```python
from build123d import *

# Parameters (mm, degrees)
SKETCH1_W            = 28
SKETCH1_H            = 45
BOSS_EXTRUDE1_DEPTH  = 7
SKETCH7_W            = 4
SKETCH7_H            = 7
BOSS_EXTRUDE2_DEPTH  = 6
SKETCH6_W            = 4
SKETCH6_H            = 7
BOSS_EXTRUDE3_DEPTH  = 6
SKETCH10_R           = 1
CUT_EXTRUDE1_DEPTH   = 6
SKETCH11_W           = 24
SKETCH11_H           = 5
CUT_EXTRUDE2_DEPTH   = 43
SKETCH16_W           = 36
SKETCH16_H           = 2
BOSS_EXTRUDE7_DEPTH  = 2
SKETCH17_W           = 36
SKETCH17_H           = 2
BOSS_EXTRUDE8_DEPTH  = 2
SKETCH30_W           = 40
SKETCH30_H           = 12
BOSS_EXTRUDE13_DEPTH = 11
SKETCH31_W           = 24
SKETCH31_H           = 10
CUT_EXTRUDE11_DEPTH  = 10
SKETCH32_W           = 24
SKETCH32_H           = 5
CUT_EXTRUDE12_DEPTH  = 1
SKETCH33_R           = 1
CUT_EXTRUDE13_DEPTH  = 11
SKETCH34_R           = 1
CUT_EXTRUDE14_DEPTH  = 11


with BuildPart() as part:
    # Sketch1 → Boss-Extrude1 (new body)
    with BuildSketch(Plane(origin=(0, 0, 0), x_dir=(1, 0, 0), z_dir=(0, 1, 0))):
        with Locations((14, 22.5)):
            Rectangle(SKETCH1_W, SKETCH1_H)
    extrude(amount=BOSS_EXTRUDE1_DEPTH)

    # Sketch7 → Boss-Extrude2 (add)
    with BuildSketch(Plane(origin=(28, 0, 0), x_dir=(0, 0, -1), z_dir=(1, 0, 0))):
        with Locations((43, 3.5)):
            Rectangle(SKETCH7_W, SKETCH7_H)
    extrude(amount=BOSS_EXTRUDE2_DEPTH)

    # Sketch6 → Boss-Extrude3 (add)
    with BuildSketch(Plane.ZY):
        with Locations((-43, 3.5)):
            Rectangle(SKETCH6_W, SKETCH6_H)
    extrude(amount=BOSS_EXTRUDE3_DEPTH)

    # Sketch10 → Cut-Extrude1 (cut)
    with BuildSketch(Plane.XY.offset(-41)):
        with Locations((-4, 2)):
            Circle(SKETCH10_R)
        with Locations((32, 2)):
            Circle(SKETCH10_R)
    extrude(amount=-CUT_EXTRUDE1_DEPTH, mode=Mode.SUBTRACT)

    # Sketch11 → Cut-Extrude2 (cut)
    with BuildSketch(Plane(origin=(0, 0, -45), x_dir=(-1, 0, 0), z_dir=(0, 0, -1))):
        with Locations((-14, 3.5)):
            Rectangle(SKETCH11_W, SKETCH11_H)
    extrude(amount=-CUT_EXTRUDE2_DEPTH, mode=Mode.SUBTRACT)

    # Sketch16 → Boss-Extrude7 (add)
    with BuildSketch(Plane.ZY):
        with Locations((-23, 4)):
            Rectangle(SKETCH16_W, SKETCH16_H)
    extrude(amount=BOSS_EXTRUDE7_DEPTH)

    # Sketch17 → Boss-Extrude8 (add)
    with BuildSketch(Plane(origin=(28, 0, 0), x_dir=(0, 0, -1), z_dir=(1, 0, 0))):
        with Locations((23, 4)):
            Rectangle(SKETCH17_W, SKETCH17_H)
    extrude(amount=BOSS_EXTRUDE8_DEPTH)

    # Sketch30 → Boss-Extrude13 (add)
    with BuildSketch(Plane(origin=(0, 0, -45), x_dir=(-1, 0, 0), z_dir=(0, 0, -1))):
        with Locations((-14, 3.5)):
            Rectangle(SKETCH30_W, SKETCH30_H)
    extrude(amount=BOSS_EXTRUDE13_DEPTH)

    # Sketch31 → Cut-Extrude11 (cut)
    with BuildSketch(Plane(origin=(0, 0, -56), x_dir=(-1, 0, 0), z_dir=(0, 0, -1))):
        with Locations((-14, 3.5)):
            Rectangle(SKETCH31_W, SKETCH31_H)
    extrude(amount=-CUT_EXTRUDE11_DEPTH, mode=Mode.SUBTRACT)

    # Sketch32 → Cut-Extrude12 (cut)
    with BuildSketch(Plane(origin=(0, 0, -46), x_dir=(-1, 0, 0), z_dir=(0, 0, -1))):
        with Locations((-14, 3.5)):
            Rectangle(SKETCH32_W, SKETCH32_H)
    extrude(amount=-CUT_EXTRUDE12_DEPTH, mode=Mode.SUBTRACT)

    # Sketch33 → Cut-Extrude13 (cut)
    with BuildSketch(Plane.XY.offset(-45)):
        with Locations((32, 2)):
            Circle(SKETCH33_R)
    extrude(amount=-CUT_EXTRUDE13_DEPTH, mode=Mode.SUBTRACT)

    # Sketch34 → Cut-Extrude14 (cut)
    with BuildSketch(Plane.XY.offset(-45)):
        with Locations((-4, 2)):
            Circle(SKETCH34_R)
    extrude(amount=-CUT_EXTRUDE14_DEPTH, mode=Mode.SUBTRACT)


solid = part.part
```
Design review of the part built by this model. Coordinates are the model's own, in mm. A direction names the side the tool comes from. Coordinates: 2 decimals unless noted, no trailing zeros. Write each loop counter-clockwise with the first axis right and the second up, starting at its lowest first coordinate (ties: lowest second). Pieces come first, ordered by that corner, then holes. Notation, with made-up numbers: M 38,19.5 L 47,19.5 A23 ccw 47,56.5 Z; hole C 79,-22.75 d3. An arc over 180 degrees is marked long. Answer as a JSON object with one key per item and string values.
Item 1: Machinability: for faces 1 (the flat face through (-1, 3, -23)), 2 (the flat face through (26, 3, -35)), 3 (the flat face through (14, -1, -45)), 4 (the flat face through (30, 4, -23)), 5 (the flat face through (-1, 4, -5)), which of the approach directions +Z, -Z, +X, -X, +Y, -Y give a long, thin tool a straight path to every point of the face, cutting with its end or side? Answer none if there is none.
Outcome:
{"face 1": "+Z, -X, -Y", "face 2": "-Z", "face 3": "+Z, +X, -X, -Y", "face 4": "+Z, +X, +Y, -Y", "face 5": "+Z, -X, +Y, -Y"}
Item 2: Draft analysis for pull direction Y (two halves, no side actions). For faces 6 (the flat face through (29, 5, -23)), 7 (the flat face through (-6, 3, -48)), 8 (the flat face through (14, -1.5, -51)), state which applies: pulls with the +Y half, pulls with the -Y half, needs draft (parallel to the pull), parting line crosses it, or undercut.
Outcome:
{"face 6": "pulls with the +Y half", "face 7": "needs draft", "face 8": "undercut"}
Item 3: Add section B-B, the plane z = -22. Give the boundary of the cut face in (x, y).
Outcome:
{"outline": "M -2,3 L 0,3 L 0,0 L 28,0 L 28,3 L 30,3 L 30,5 L 28,5 L 28,7 L 0,7 L 0,5 L -2,5 Z; hole M 2,1 L 26,1 L 26,6 L 2,6 Z"}
Item 4: Wall thickness on probe 1 along X at (y, z) = (2.25, -11.5); probe 2 along Y at (x, z) = (9.5, -3); probe 3 along Y at (x, z) = (32, -46.5): over which ranges is each line inside the solid? List them lowest first.
Outcome:
{"probe 1": "0 to 2, 26 to 28", "probe 2": "0 to 1, 6 to 7", "probe 3": "-2.5 to 1, 3 to 9.5"}
Item 5: Add section C-C, the plane y = 2. Give the boundary of the cut face in (x, z).
Outcome:
{"outline": "M -6,-56 L -5,-56 L -5,-41 L -6,-41 Z; M -3,-56 L 2,-56 L 2,-2 L 26,-2 L 26,-56 L 31,-56 L 31,-41 L 28,-41 L 28,0 L 0,0 L 0,-41 L -3,-41 Z; M 33,-56 L 34,-56 L 34,-41 L 33,-41 Z"}
Item 6: Insertion check: pin 1 Ø1.5 at (x, z) = (15.5, -37.5) entering from +Y; pin 2 Ø3 at (x, y) = (32, 2) entering from -Z; pin 3 Ø0.6 at (y, z) = (3.5, -30.5) entering from -X; pin 4 Ø2 at (x, z) = (-0.5, -23.5) entering from -Y. Each pin has a flat end and moves straight along its axis. Give the tip position at first contact, or say it passes through.
Outcome:
{"pin 1": "y = 7", "pin 2": "z = -56", "pin 3": "x = -2", "pin 4": "y = 0"}
Item 7: Add section D-D, the plane x = 24. Give the boundary of the cut face in (y, z), and give its area (3 significant figures).
Outcome:
{"outline": "M -2.5,-56 L -1.5,-56 L -1.5,-46 L 1,-46 L 1,-2 L 6,-2 L 6,-46 L 8.5,-46 L 8.5,-56 L 9.5,-56 L 9.5,-45 L 7,-45 L 7,0 L 0,0 L 0,-45 L -2.5,-45 Z", "area": "127 mm²"}
Item 8: Add section A-A, the plane x = -4. Give the boundary of the cut face in (y, z), and give its area (3 significant figures).
Outcome:
{"outline": "M -2.5,-56 L 1,-56 L 1,-41 L 0,-41 L 0,-45 L -2.5,-45 Z; M 3,-56 L 9.5,-56 L 9.5,-45 L 7,-45 L 7,-41 L 3,-41 Z", "area": "130 mm²"}
